Model file for the job. Use its own axes, mm. Coordinates: 2 decimals unless noted, no trailing zeros. Loops run counter-clockwise (first coordinate to the right, second up) from the corner with the lowest first, then second, coordinate; pieces in that order, holes last. Notation, with made-up numbers: (-37.5, -20.75) - (-14.5, -20.75) arc R29 ccw to (-14.5, 16.25) - close; hole circle Ø7 at (5.5, 9.5). An arc over 180 degrees is marked (long way). Write each question's results on one line, items separated by ' | '. Start each with the question number.
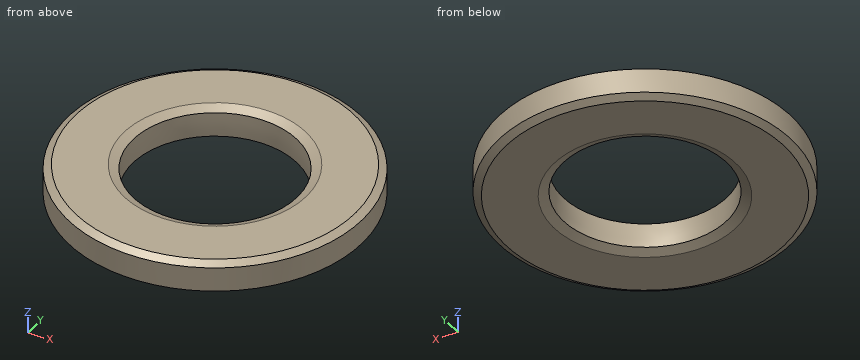
```python
from build123d import *
from OCP.BRepFilletAPI import BRepFilletAPI_MakeChamfer

# Parameters (mm, degrees)
BOSS_EXTRUDE1_DEPTH      = 1
BOSS_EXTRUDE1_DEPTH_BACK = 1
SKETCH3_R                = 9
SKETCH3_R_2              = 5
CHAMFER1_SIZE            = 0.254
CHAMFER1_SIZE2           = 0.439940905
CHAMFER2_SIZE            = 0.536952942


with BuildPart() as part:
    # Sketch3 → Boss-Extrude1 (new, two sides: drawn at the far end of the back side and taken through both)
    with BuildSketch(Plane.XY.offset(-BOSS_EXTRUDE1_DEPTH_BACK)):
        Circle(SKETCH3_R)
        Circle(SKETCH3_R_2, mode=Mode.SUBTRACT)
    extrude(amount=BOSS_EXTRUDE1_DEPTH + BOSS_EXTRUDE1_DEPTH_BACK)

    # Chamfer1: one chamfer whose edges measure the first distance from different faces: ONE call of the kernel's chamfer builder (chamfer() names one face for all edges)
    chamfer1_edges_1 = [part.edges().sort_by_distance(p)[0] for p in [
        (-9, 0, 1),
    ]]
    chamfer1_side_1 = [part.faces().sort_by_distance(p)[0] for p in [
        (-9, 0, 0.5),
    ]]
    chamfer1_edges_2 = [part.edges().sort_by_distance(p)[0] for p in [
        (-9, 0, -1),
    ]]
    chamfer1_side_2 = [part.faces().sort_by_distance(p)[0] for p in [
        (-9, 0, -0.5),
    ]]
    chamfer1 = BRepFilletAPI_MakeChamfer(part.part.solid().wrapped)
    for e in chamfer1_edges_1:
        chamfer1.Add(CHAMFER1_SIZE, CHAMFER1_SIZE2, e.wrapped, chamfer1_side_1[0].wrapped)  # the first distance lies on this face
    for e in chamfer1_edges_2:
        chamfer1.Add(CHAMFER1_SIZE, CHAMFER1_SIZE2, e.wrapped, chamfer1_side_2[0].wrapped)  # the first distance lies on this face
    add(Compound.cast(chamfer1.Shape()), mode=Mode.REPLACE)

    # Sketch4 → Cut-Revolve1 (revolve, cut)
    with BuildSketch(Plane(origin=(0, 0, 0), x_dir=(0, 0, -1), z_dir=(1, 0, 0)), mode=Mode.PRIVATE) as cut_revolve1_sk:
        with BuildLine():
            Line((-1, 4.9492), (-1, 5.0508))
            ThreePointArc((-1, 5.0508), (0, 5), (1, 5.0508))
            Line((1, 5.0508), (1, 4.9492))
            Line((1, 4.9492), (-1, 4.9492))
        make_face()
    revolve(cut_revolve1_sk.sketch.rotate(Axis((0, 0, 1), (0, 0, -1)), 90), axis=Axis((0, 0, 1), (0, 0, -1)), mode=Mode.SUBTRACT)

    # Chamfer2
    # the kernel refuses this chamfer: 0.536952942, 0.254 mm, written as the material it takes off along each edge
    with BuildSketch(Plane(origin=(0, 0, -1), x_dir=(1, 0, 0), z_dir=(0, 1, 0))) as chamfer2_piece_1:
        with BuildLine():
            Line((5.0508 + CHAMFER2_SIZE, 0), (5.028453739, -0.251168371))
            ThreePointArc((5.028453739, -0.251168371), (5.038361074, -0.130738), (5.0508, 0))
            Line((5.0508, 0), (5.0508 + CHAMFER2_SIZE, 0))
        make_face()
    revolve(axis=Axis((0, 0, -1), (0, 0, -1)), mode=Mode.SUBTRACT)
    with BuildSketch(Plane(origin=(0, 0, 1), x_dir=(1, 0, 0), z_dir=(0, 1, 0))) as chamfer2_piece_2:
        with BuildLine():
            Line((5.0508 + CHAMFER2_SIZE, 0), (5.028453739, 0.251168371))
            ThreePointArc((5.028453739, 0.251168371), (5.038361074, 0.130738), (5.0508, 0))
            Line((5.0508, 0), (5.0508 + CHAMFER2_SIZE, 0))
        make_face()
    revolve(axis=Axis((0, 0, 1), (0, 0, -1)), mode=Mode.SUBTRACT)


solid = part.part
```
Q1. Cut at C-C (z = 0.3). List the corners of the cut face in (x, y), and give its area (3 significant figures).
Q2. Drill centre lines: L1, parallel to X at y = 3.75, z = 0; L2, parallel to X at y = -3.25, z = 0; L3, parallel to Y at x = -0.5, z = -0.15. Where is each one in solid material? Low to high. Write a range as from..to.
Q3. Pin check, flat tips, straight feed: pin 1 (4 mm diameter, centred on x = 1, y = -2, fed in from +Z); pin 2 (1 mm diameter, centred on y = -7, z = -0.5, fed in from +X); pin 3 (10 mm diameter, centred on x = 1.5, y = 1, fed in from -Z). Stop position of each tip, or through.
Q4. Cut at A-A (x = 0). List the corners of the cut face in (y, z), and give its area (3 significant figures).
Check result:
1) outline: circle Ø18 at (0, 0); hole circle Ø10.01 at (0, 0) | area: 176 mm²
2) L1: -8.18..-3.31, 3.31..8.18 | L2: -8.39..-3.8, 3.8..8.39 | L3: -8.99..-4.98, 4.98..8.99
3) pin 1: through | pin 2: x = 6.22 | pin 3: z = -1
4) outline: (-9, -0.75) - (-8.56, -1) - (-5.59, -1) - (-5.03, -0.75) arc R9.87 ccw to (-5.03, 0.75) - (-5.59, 1) - (-8.56, 1) - (-9, 0.75) - close; (5.03, -0.75) - (5.59, -1) - (8.56, -1) - (9, -0.75) - (9, 0.75) - (8.56, 1) - (5.59, 1) - (5.03, 0.75) arc R9.87 ccw to start | area: 15.4 mm²
